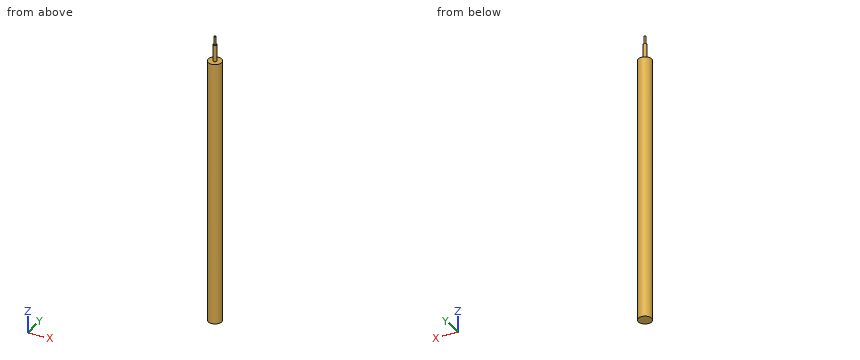
from build123d import *

# Parameters (mm, degrees)
SKETCH1_R           = 4
BOSS_EXTRUDE1_DEPTH = 160
SKETCH2_R           = 1
SKETCH2_R_2         = 0.5
BOSS_EXTRUDE2_DEPTH = 10
SKETCH2_3_R         = 0.5
BOSS_EXTRUDE3_DEPTH = 15


with BuildPart() as part:
    # Sketch1 → Boss-Extrude1 (new body)
    with BuildSketch(Plane.XY):
        Circle(SKETCH1_R)
    extrude(amount=BOSS_EXTRUDE1_DEPTH)

    # Sketch2 → Boss-Extrude2 (add)
    # profile 1 of 2: a face of its own
    with BuildSketch(Plane.XY.offset(160)):
        Circle(SKETCH2_R)
        Circle(SKETCH2_R_2, mode=Mode.SUBTRACT)
    # profile 2 of 2: a face of its own
    with BuildSketch(Plane.XY.offset(160)):
        Circle(SKETCH2_R_2)
    extrude(amount=BOSS_EXTRUDE2_DEPTH)

    # Sketch2_3 → Boss-Extrude3 (add)
    with BuildSketch(Plane.XY.offset(160)):
        Circle(SKETCH2_3_R)
    extrude(amount=BOSS_EXTRUDE3_DEPTH)


solid = part.part
The model under review builds one solid part; all positions refer to its coordinate system, in mm. Round coordinates to 2 decimals unless told otherwise and drop trailing zeros. Loops run counter-clockwise (first coordinate to the right, second up) from the corner with the lowest first, then second, coordinate; pieces in that order, holes last. Notation, with made-up numbers: (25.25, -11.75) -> (55.25, -11.75) arc R27 cw to (55.25, 8.25) -> close; hole circle Ø10 at (49.5, -22.5). An arc over 180 degrees is marked (long way). One line per question, with ' | ' between items. Start each with the question number.
Item 1: For pin 1 (1.5 mm diameter, centred on y = -0.5, z = 54, fed in from +X); pin 2 (4 mm diameter, centred on x = 2.5, z = 137.5, fed in from -Y); pin 3 (3 mm diameter, centred on x = -2.5, y = -1, fed in from +Z); pin 4 (1.5 mm diameter, centred on x = 2.5, z = 101, fed in from +Y), all flat-tipped, find the tip position at first contact; note any pin that passes through.
Item 2: Add section A-A, the plane z = 29. Write out the cut boundary in (x, y).
Item 3: Add section B-B, the plane y = -2.5. Write out the cut boundary in (x, z), then the cut area to 3 significant figures.
Item 4: Wall thickness on line 1 along Z through (x, y) = (-2.5, -0.5); line 2 along X through (y, z) = (-0.5, 126.5); line 3 along Y through (x, z) = (-0.25, 116.5): over which ranges is each line inside the solid? List them lowest first. Write a range as [from, to].
Return value:
1) pin 1: stops at x = 4 | pin 2: stops at y = -3.97 | pin 3: stops at z = 160 | pin 4: stops at y = 3.6
2) outline: circle Ø8 at (0, 0)
3) outline: (-3.12, 0) -> (3.12, 0) -> (3.12, 160) -> (-3.12, 160) -> close | area: 999 mm2
4) line 1: z = [0, 160] | line 2: x = [-3.97, 3.97] | line 3: y = [-3.99, 3.99]
